Autodesk Fusion 360 part; units mm, degrees
sketch "Sketch1" plane through (0, 0, 0) normal (0, 0, 1) x (1, 0, 0)
  line L0 (0, 0) -> (74, 0)
  line L1 (74, 0) -> (74, 28)
  line L2 (74, 28) -> (0, 28)
  line L3 (0, 28) -> (0, 0)
  dimension "d1" = 74
  dimension "d2" = 28
extrude "Extrude1" add sketch "Sketch1" along normal blind 2
sketch "Sketch2" plane through (0, 0, 2) normal (0, 0, 1) x (-1, 0, 0)
  line L0 (0, -28) -> (0, 0)
  line L1 (0, 0) -> (-74, 0)
  line L2 (-74, 0) -> (-74, -28)
  line L3 (-74, -28) -> (0, -28)
  line L4 (-3, -24.5) -> (-71, -24.5)
  line L5 (-71, -24.5) -> (-71, -3.5)
  line L6 (-71, -3.5) -> (-3, -3.5)
  line L7 (-3, -3.5) -> (-3, -24.5)
  dimension "d5" = 3.5
  dimension "d6" = 3
  dimension "d7" = 3.5
  dimension "d8" = 3
extrude "Extrude2" cut sketch "Sketch2" against normal blind 2 contours L4 L5 L6 L7
fillet "Fillet1" radius 2 4 edges at (74, 0, 1) (74, 28, 1) (0, 28, 1) (0, 0, 1)
fillet "Fillet2" radius 1 4 edges at (71, 24.5, 1) (3, 24.5, 1) (3, 3.5, 1) (71, 3.5, 1)
chamfer "Chamfer1" distance 1 angle 45 8 edges at (3.2929, 3.7929, 2) (3, 14, 2) (3.2929, 24.2071, 2) (37, 24.5, 2) (70.7071, 24.2071, 2) (71, 14, 2) (70.7071, 3.7929, 2) (37, 3.5, 2)
Here's how the part is built. I have some questions about the finished solid (model axes, mm). A direction names the side the tool comes from. Round coordinates to 2 decimals unless told otherwise and drop trailing zeros. Order: outer loops, then holes, each group sorted by start corner. A loop starts at its lowest first (then second) coordinate and runs counter-clockwise, first axis right, second up. Notation, with made-up numbers: M -39.75,-5 L -31.75,-5 A25 cw -31.75,13 Z; hole C 8,38 d11. An arc over 180 degrees is marked long. Answer in a Markdown table with one row per item.
Item 1: Thinking about a two-plate mould opening in Y: for faces 3 (the face through (37, 0, 1)), 4 (the face through (3, 3.52, 1.4)), 5 (the face through (0.6, 27.43, 1.01)), 6 (the face through (70.98, 3.5, 1.4)), which applies, +Y half, -Y half, draft (parallel to the pull), parting line (faces both ways), or undercut?
A:
| item | result |
|---|---|
| face 3 | -Y half |
| face 4 | undercut |
| face 5 | +Y half |
| face 6 | undercut |
Item 2: Imagine slicing it at B-B, the plane x = 61. Write out the boundary of the cut face in (y, z).
A:
| item | result |
|---|---|
| outline | M 0,0 L 3.5,0 L 3.5,1 L 2.5,2 L 0,2 Z; M 24.5,0 L 28,0 L 28,2 L 25.5,2 L 24.5,1 Z |
Item 3: Imagine slicing it at A-A, the plane y = 21.75. Write out the boundary of the cut face in (x, z), and give its area (3 significant figures).
A:
| item | result |
|---|---|
| outline | M 0,0 L 3,0 L 3,1 L 2,2 L 0,2 Z; M 71,0 L 74,0 L 74,2 L 72,2 L 71,1 Z |
| area | 11.0 mm2 |
Item 4: For faces 1 (the face through (74, 14, 1)), 2 (the face through (71, 24.48, 1.4)), which set-ups out of +Z, -Z, +X, -X, +Y, -Y let a thin tool reach every point of the face, with its end or its side?
A:
| item | result |
|---|---|
| face 1 | +Z, -Z, +X, +Y, -Y |
| face 2 | +Z |
Item 5: Imagine slicing it at C-C, the plane z = 1.5. Write out the boundary of the cut face in (x, y), and give its area (3 significant figures).
A:
| item | result |
|---|---|
| outline | M 0,2 A2 ccw 2,0 L 72,0 A2 ccw 74,2 L 74,26 A2 ccw 72,28 L 2,28 A2 ccw 0,26 Z; hole M 2.5,4.5 A1.5 ccw 4,3 L 70,3 A1.5 ccw 71.5,4.5 L 71.5,23.5 A1.5 ccw 70,25 L 4,25 A1.5 ccw 2.5,23.5 Z |
| area | 552 mm2 |
Item 6: If I drill on L1, parallel to Y at x = 35, z = 0.65; L2, parallel to X at y = 13.5, z = 0.1; L3, parallel to X at y = 22.5, z = 1.25, over which ranges is the centre line in solid material (lowest first)? Write a range as from..to.
A:
| item | result |
|---|---|
| L1 | y = 0..3.5, 24.5..28 |
| L2 | x = 0..3, 71..74 |
| L3 | x = 0..2.75, 71.25..74 |
Item 7: I'm going to push a flat-ended pin straight in: pin 1 (1.5 mm diameter, centred on x = 15.5, y = 4.5, fed in from -Z). Where does the tip first touch, or does it pass through?
A:
| item | result |
|---|---|
| pin 1 | passes through |
